```python
from build123d import *

# Parameters (mm, degrees)
BOSS_EXTRUDE1_DEPTH      = 3
BOSS_EXTRUDE1_DEPTH_BACK = 3
FILLET1_R                = 1


with BuildPart() as part:
    # Sketch1 → Boss-Extrude1 (new, two sides: drawn at the far end of the back side and taken through both)
    with BuildSketch(Plane.XY.offset(-BOSS_EXTRUDE1_DEPTH_BACK)):
        Polygon((-6, 0), (0, 0), (0, 4.5), (-3, 4.5), (-3, 1.5), (-4.5, 1.5), align=None)
        Polygon((0, 0), (6, 0), (4.5, 1.5), (3, 1.5), (3, 4.5), (0, 4.5), align=None)
    extrude(amount=BOSS_EXTRUDE1_DEPTH + BOSS_EXTRUDE1_DEPTH_BACK)

    # Sketch2 → Cut-Revolve1 (revolve, cut)
    with BuildSketch(Plane(origin=(0, 0, 0), x_dir=(0, 0, -1), z_dir=(1, 0, 0))):
        with BuildLine():
            Line((0, 0.4), (0, 5.6))
            ThreePointArc((0, 5.6), (-2.6, 3), (0, 0.4))
        make_face()
    revolve(axis=Axis((0, 0.4, 0), (0, 1, 0)), mode=Mode.SUBTRACT)

    # Fillet1
    # the kernel refuses this fillet: 1 mm, written as the material it adds along each edge
    with BuildSketch(Plane(origin=(-3, 1.5, 3), x_dir=(-1, 0, 0), z_dir=(0, 0, -1)), Plane(origin=(3, 1.5, -3), x_dir=(1, 0, 0), z_dir=(0, 0, 1))) as fillet1_piece_1:
        with BuildLine():
            CenterArc((FILLET1_R, FILLET1_R), FILLET1_R, 180, 90)
            Line((0, FILLET1_R), (0, 0))
            Line((0, 0), (FILLET1_R, 0))
        make_face()
    extrude(amount=6)
    # the kernel refuses this fillet: 1 mm, written as the material it takes off along each edge
    with BuildSketch(Plane(origin=(-2, 3.5, -2), x_dir=(-1, 0, 0), z_dir=(0, 1, 0))) as fillet1_2_piece_1_section:
        Polygon((0, 0), (FILLET1_R, 0), (FILLET1_R, -FILLET1_R), (0, -FILLET1_R), align=None)
    fillet1_2_piece_1 = extrude(amount=FILLET1_R, mode=Mode.PRIVATE)
    fillet1_2_piece_1 = fillet1_2_piece_1 - Plane(origin=(-2, 3.5, -2), x_dir=(0.7071067811865475, 0, 0.7071067811865475), z_dir=(0, 1, 0)) * Sphere(FILLET1_R, mode=Mode.PRIVATE)
    add(fillet1_2_piece_1, mode=Mode.SUBTRACT)
    with BuildSketch(Plane(origin=(-2, 3.5, 2), x_dir=(-1, 0, 0), z_dir=(0, 1, 0))) as fillet1_2_piece_2_section:
        Polygon((0, 0), (FILLET1_R, 0), (FILLET1_R, FILLET1_R), (0, FILLET1_R), align=None)
    fillet1_2_piece_2 = extrude(amount=FILLET1_R, mode=Mode.PRIVATE)
    fillet1_2_piece_2 = fillet1_2_piece_2 - Plane(origin=(-2, 3.5, 2), x_dir=(0.7071067811865475, 0, -0.7071067811865475), z_dir=(0, 1, 0)) * Sphere(FILLET1_R, mode=Mode.PRIVATE)
    add(fillet1_2_piece_2, mode=Mode.SUBTRACT)
    with BuildSketch(Plane(origin=(2, 3.5, -2), x_dir=(0, 0, -1), z_dir=(0, 1, 0))) as fillet1_2_piece_3_section:
        Polygon((0, 0), (FILLET1_R, 0), (FILLET1_R, -FILLET1_R), (0, -FILLET1_R), align=None)
    fillet1_2_piece_3 = extrude(amount=FILLET1_R, mode=Mode.PRIVATE)
    fillet1_2_piece_3 = fillet1_2_piece_3 - Plane(origin=(2, 3.5, -2), x_dir=(-0.7071067811865475, 0, 0.7071067811865475), z_dir=(0, 1, 0)) * Sphere(FILLET1_R, mode=Mode.PRIVATE)
    add(fillet1_2_piece_3, mode=Mode.SUBTRACT)
    with BuildSketch(Plane(origin=(2, 3.5, 2), x_dir=(0, 0, 1), z_dir=(0, 1, 0))) as fillet1_2_piece_4_section:
        Polygon((0, 0), (FILLET1_R, 0), (FILLET1_R, FILLET1_R), (0, FILLET1_R), align=None)
    fillet1_2_piece_4 = extrude(amount=FILLET1_R, mode=Mode.PRIVATE)
    fillet1_2_piece_4 = fillet1_2_piece_4 - Plane(origin=(2, 3.5, 2), x_dir=(-0.7071067811865475, 0, -0.7071067811865475), z_dir=(0, 1, 0)) * Sphere(FILLET1_R, mode=Mode.PRIVATE)
    add(fillet1_2_piece_4, mode=Mode.SUBTRACT)
    with BuildSketch(Plane(origin=(7, 1.5, -3), x_dir=(0, -1, 0), z_dir=(-1, 0, 0)), Plane(origin=(-4, 1.5, -3), x_dir=(0, -1, 0), z_dir=(-1, 0, 0))) as fillet1_2_piece_5:
        with BuildLine():
            CenterArc((FILLET1_R, FILLET1_R), FILLET1_R, 180, 90)
            Line((0, FILLET1_R), (0, 0))
            Line((0, 0), (FILLET1_R, 0))
        make_face()
    extrude(amount=3, mode=Mode.SUBTRACT)
    with BuildSketch(Plane(origin=(-4.5, 1.5, 4.035533906), x_dir=(-0.7071067811865516, -0.7071067811865435, 0), z_dir=(0, 0, -1)), Plane(origin=(4.5, 1.5, -4.035533906), x_dir=(0.707106781186551, -0.707106781186544, 0), z_dir=(0, 0, 1))) as fillet1_2_piece_6:
        with BuildLine():
            CenterArc((FILLET1_R * 0.414213562373, -FILLET1_R), FILLET1_R, 90, 45)
            Line((-FILLET1_R * 0.292893218813, -FILLET1_R * 0.292893218813), (0, 0))
            Line((0, 0), (FILLET1_R * 0.414213562373, 0))
        make_face()
    extrude(amount=8.071067812, mode=Mode.SUBTRACT)
    with BuildSketch(Plane(origin=(-3, 4.5, -2), x_dir=(1, 0, 0), z_dir=(0, 0, 1)), Plane(origin=(3, 4.5, -2), x_dir=(0, -1, 0), z_dir=(0, 0, 1)), Plane(origin=(-2, 4.5, -3), x_dir=(0, -1, 0), z_dir=(1, 0, 0)), Plane(origin=(2, 4.5, 3), x_dir=(0, -1, 0), z_dir=(-1, 0, 0))) as fillet1_2_piece_7:
        with BuildLine():
            CenterArc((FILLET1_R, -FILLET1_R), FILLET1_R, 90, 90)
            Line((0, -FILLET1_R), (0, 0))
            Line((0, 0), (FILLET1_R, 0))
        make_face()
    extrude(amount=4, mode=Mode.SUBTRACT)
    with BuildSketch(Plane(origin=(3, 2.5, -3), x_dir=(-1, 0, 0), z_dir=(0, 1, 0)), Plane(origin=(-3, 3.5, -3), x_dir=(1, 0, 0), z_dir=(0, -1, 0))) as fillet1_2_piece_8:
        with BuildLine():
            CenterArc((FILLET1_R, FILLET1_R), FILLET1_R, 180, 90)
            Line((0, FILLET1_R), (0, 0))
            Line((0, 0), (FILLET1_R, 0))
        make_face()
    extrude(amount=1, mode=Mode.SUBTRACT)
    with BuildSketch(Plane(origin=(-3, 3.5, 3), x_dir=(1, 0, 0), z_dir=(0, -1, 0)), Plane(origin=(3, 2.5, 3), x_dir=(-1, 0, 0), z_dir=(0, 1, 0))) as fillet1_2_piece_9:
        with BuildLine():
            CenterArc((FILLET1_R, -FILLET1_R), FILLET1_R, 90, 90)
            Line((0, -FILLET1_R), (0, 0))
            Line((0, 0), (FILLET1_R, 0))
        make_face()
    extrude(amount=1, mode=Mode.SUBTRACT)
    with BuildSketch(Plane(origin=(-4, 1.5, 3), x_dir=(0, -1, 0), z_dir=(-1, 0, 0)), Plane(origin=(7, 1.5, 3), x_dir=(0, -1, 0), z_dir=(-1, 0, 0))) as fillet1_2_piece_10:
        with BuildLine():
            CenterArc((FILLET1_R, -FILLET1_R), FILLET1_R, 90, 90)
            Line((0, -FILLET1_R), (0, 0))
            Line((0, 0), (FILLET1_R, 0))
        make_face()
    extrude(amount=3, mode=Mode.SUBTRACT)
    with BuildSketch(Plane(origin=(-4, 2.5, -3), x_dir=(0, -1, 0), z_dir=(-1, 0, 0))) as fillet1_2_piece_11:
        with BuildLine():
            CenterArc((1 + FILLET1_R, FILLET1_R), FILLET1_R, 180, 90)
            Line((1, FILLET1_R), (1, 0))
            Line((1, 0), (1 + FILLET1_R, 0))
        make_face()
    revolve(axis=Axis((-4, 2.5, -3), (0, 0, 1)), revolution_arc=90, mode=Mode.SUBTRACT)
    with BuildSketch(Plane(origin=(4, 2.5, 3), x_dir=(0, -1, 0), z_dir=(1, 0, 0))) as fillet1_2_piece_12:
        with BuildLine():
            CenterArc((1 + FILLET1_R, FILLET1_R), FILLET1_R, 180, 90)
            Line((1, FILLET1_R), (1, 0))
            Line((1, 0), (1 + FILLET1_R, 0))
        make_face()
    revolve(axis=Axis((4, 2.5, 3), (0, 0, -1)), revolution_arc=90, mode=Mode.SUBTRACT)
    with BuildSketch(Plane(origin=(-4, 2.5, 3), x_dir=(0, -1, 0), z_dir=(-1, 0, 0))) as fillet1_2_piece_13:
        with BuildLine():
            CenterArc((1 + FILLET1_R, -FILLET1_R), FILLET1_R, 90, 90)
            Line((1, -FILLET1_R), (1, 0))
            Line((1, 0), (1 + FILLET1_R, 0))
        make_face()
    revolve(axis=Axis((-4, 2.5, 3), (0, 0, 1)), revolution_arc=90, mode=Mode.SUBTRACT)
    with BuildSketch(Plane(origin=(4, 2.5, -3), x_dir=(0, -1, 0), z_dir=(1, 0, 0))) as fillet1_2_piece_14:
        with BuildLine():
            CenterArc((1 + FILLET1_R, -FILLET1_R), FILLET1_R, 90, 90)
            Line((1, -FILLET1_R), (1, 0))
            Line((1, 0), (1 + FILLET1_R, 0))
        make_face()
    revolve(axis=Axis((4, 2.5, -3), (0, 0, -1)), revolution_arc=90, mode=Mode.SUBTRACT)


solid = part.part
```
Could you check a few things on this model? Use its own coordinates, in mm. A direction names the side the tool comes from. Round coordinates to 2 decimals unless told otherwise and drop trailing zeros. Loops run counter-clockwise (first coordinate to the right, second up) from the corner with the lowest first, then second, coordinate; pieces in that order, holes last. Notation, with made-up numbers: (6, 28) - (11, 28) arc R15 ccw to (11, 56) - close; hole circle Ø8 at (20.25, 4). An arc over 180 degrees is marked (long way). Answer in a Markdown table with one row per item. Add a question column.
(1) I need wall thicknesses on line 1 along Z through (x, y) = (2.25, 3.7); line 2 along X through (y, z) = (2.7, 0.5); line 3 along X through (y, z) = (2.55, 2.25). Which ranges of each line are inside material? Lowest first, please.
(2) If we section it at B-B (z = 2.25): Please give me the cut outline in (x, y), plus the area to 3 significant figures.
(3) If we section it at D-D (z = 1.25): Please give me the cut outline in (x, y).
(4) I'm going to push flat-ended pins straight in: pin 1 (2 mm diameter, centred on x = 2.5, y = 2, fed in from -Z); pin 2 (0.5 mm diameter, centred on y = 3, z = 1, fed in from -X); pin 3 (0.8 mm diameter, centred on y = 3, z = -0.5, fed in from +X); pin 4 (2 mm diameter, centred on y = 2, z = -1, fed in from +X). Where does each tip first touch, or does it pass through?
(5) If we section it at C-C (x = -1.5): Please give me the cut outline in (y, z), plus the area to 3 significant figures.
(6) For faces 1 (the face through (2.699, 2.993, 2.715)), 2 (the face through (1.7, 4.5, 1.7)), 3 (the face through (-4.6, 1.1, 2.8)), 4 (the face through (-4.4, 1.1, -2.8)), 5 (the face through (3, 3, 0)), which set-ups out of +Z, -Z, +X, -X, +Y, -Y let a thin tool reach every point of the face, with its end or its side?
(7) If we section it at A-A (y = 3): Please give me the cut outline in (x, z), plus the area to 3 significant figures.
Model answer:
| question | item | result |
|---|---|---|
| 1 | line 1 | z = -2.95 to -1.1, 1.1 to 2.95 |
| 1 | line 2 | x = -3 to -2.53, 2.53 to 3 |
| 1 | line 3 | x = -2.97 to -1.22, 1.22 to 2.97 |
| 2 | outline | (-6, 0) - (6, 0) - (4.79, 1.21) arc R1 ccw to (4.34, 1.47) - (4, 1.47) arc R1.03 cw to (2.97, 2.5) - (2.97, 3.5) arc R0.97 ccw to (2, 4.47) - (-2, 4.47) arc R0.97 ccw to (-2.97, 3.5) - (-2.97, 2.5) arc R1.03 cw to (-4, 1.47) - (-4.34, 1.47) arc R1 ccw to (-4.79, 1.21) - close; hole circle Ø2.61 at (0, 3) |
| 2 | area | 28.0 mm² |
| 3 | outline | (-6, 0) - (6, 0) - (4.79, 1.21) arc R1 ccw to (4.09, 1.5) - (4, 1.5) arc R1 cw to (3, 2.5) - (3, 3.5) arc R1 ccw to (2, 4.5) - (1.72, 4.5) arc R2.28 cw (long way) to (-1.72, 4.5) - (-2, 4.5) arc R1 ccw to (-3, 3.5) - (-3, 2.5) arc R1 cw to (-4, 1.5) - (-4.09, 1.5) arc R1 ccw to (-4.79, 1.21) - close |
| 4 | pin 1 | stops at z = -3 |
| 4 | pin 2 | stops at x = -3 |
| 4 | pin 3 | stops at x = 3 |
| 4 | pin 4 | stops at x = 5 |
| 5 | outline | (0, -3) - (3.5, -3) arc R1 ccw to (4.5, -2) - (4.5, -1.5) arc R2.12 cw (long way) to (4.5, 1.5) - (4.5, 2) arc R1 ccw to (3.5, 3) - (0, 3) - close |
| 5 | area | 13.7 mm² |
| 6 | face 1 | +Z, +X, +Y |
| 6 | face 2 | +Z, -Z, +X, -X, +Y |
| 6 | face 3 | +Z, -X, +Y |
| 6 | face 4 | -Z, -X, +Y |
| 6 | face 5 | +Z, -Z, +X, +Y |
| 7 | outline | (-3, -2) arc R1 ccw to (-2, -3) - (2, -3) arc R1 ccw to (3, -2) - (3, 2) arc R1 ccw to (2, 3) - (-2, 3) arc R1 ccw to (-3, 2) - close; hole circle Ø5.2 at (0, 0) |
| 7 | area | 13.9 mm² |
